```python
from build123d import *

# Parameters (mm, degrees)
SKETCH1_W           = 165
SKETCH1_H           = 107
BOSS_EXTRUDE1_DEPTH = 10
SKETCH2_W           = 9
SKETCH2_H           = 9
CUT_EXTRUDE1_DEPTH  = 5
SKETCH3_W           = 17.586391164
SKETCH3_H           = 24.095664715
CUT_EXTRUDE2_DEPTH  = 5
SKETCH6_W           = 10.5
SKETCH6_H           = 16
CUT_EXTRUDE3_DEPTH  = 130.934107916
SKETCH8_R           = 3.05
CUT_EXTRUDE4_DEPTH  = 130.934107916
SKETCH9_W           = 9
SKETCH9_H           = 9
CUT_EXTRUDE5_DEPTH  = 5


with BuildPart() as part:
    # Sketch1 → Boss-Extrude1 (new body)
    with BuildSketch(Plane.XY):
        with BuildLine():
            Line((-106.68, 73.5), (-31.75, 73.5))
            ThreePointArc((-31.75, 73.5), (0, 58.078932216), (31.75, 73.5))
            Line((31.75, 73.5), (106.68, 73.5))
            Line((106.68, 73.5), (97.79, -63.5))
            Line((97.79, -63.5), (-97.79, -63.5))
            Line((-97.79, -63.5), (-106.68, 73.5))
        make_face()
        Rectangle(SKETCH1_W, SKETCH1_H, mode=Mode.SUBTRACT)
    extrude(amount=BOSS_EXTRUDE1_DEPTH)

    # Sketch2 → Cut-Extrude1 (cut)
    with BuildSketch(Plane.XY.offset(10)):
        with Locations((78, 58)):
            Rectangle(SKETCH2_W, SKETCH2_H)
        with Locations((-78, 58)):
            Rectangle(SKETCH2_W, SKETCH2_H)
    extrude(amount=-CUT_EXTRUDE1_DEPTH, mode=Mode.SUBTRACT)

    # Sketch3 → Cut-Extrude2 (cut)
    with BuildSketch(Plane.XY.offset(10)):
        with Locations((-91.293195582, 41.716713566)):
            Rectangle(SKETCH3_W, SKETCH3_H)
    extrude(amount=-CUT_EXTRUDE2_DEPTH, mode=Mode.SUBTRACT)

    # Sketch6 → Cut-Extrude3 (cut, through all)
    with BuildSketch(Plane(origin=(0, 0, 0), x_dir=(-1, 0, 0), z_dir=(0, 0, -1))):
        with Locations((92.403067071, 12.157965544)):
            Rectangle(SKETCH6_W, SKETCH6_H)
    extrude(amount=-CUT_EXTRUDE3_DEPTH, mode=Mode.SUBTRACT)

    # Sketch8 → Cut-Extrude4 (cut, through all)
    with BuildSketch(Plane(origin=(0, 0, 0), x_dir=(-1, 0, 0), z_dir=(0, 0, -1))):
        with Locations((91.642033661, -12.875359706)):
            Circle(SKETCH8_R)
    extrude(amount=-CUT_EXTRUDE4_DEPTH, mode=Mode.SUBTRACT)

    # Sketch9 → Cut-Extrude5 (cut)
    with BuildSketch(Plane.XY.offset(10)):
        with Locations((78, -58)):
            Rectangle(SKETCH9_W, SKETCH9_H)
        with Locations((-78, -58)):
            Rectangle(SKETCH9_W, SKETCH9_H)
    extrude(amount=-CUT_EXTRUDE5_DEPTH, mode=Mode.SUBTRACT)


solid = part.part
```
Geometry: final body of the model. Coordinates: model frame, mm. A direction names the side the tool comes from. Round coordinates to 2 decimals unless told otherwise and drop trailing zeros. Write each loop counter-clockwise with the first axis right and the second up, starting at its lowest first coordinate (ties: lowest second). Pieces come first, ordered by that corner, then holes.
Item 1: Section query A-A (x = -77). Return loops of the section in (y, z), plus the area to 3 significant figures.
Item 2: Section query D-D (y = 43). Return loops of the section in (x, z), plus the area to 3 significant figures.
Item 3: Pin query (flat end, axial travel): P1, Ø1.5, axis at y = -58.5, z = 7, coming from the +X side; P2, Ø2.5, axis at y = -57.5, z = 7, coming from the -X side; P3, Ø4, axis at y = 3.5, z = 8, coming from the +X side. Return the tip coordinate at first contact, or that it passes through.
Item 4: Mould query, pull axis Y, two halves, no side actions, for faces 4 (the face through (-70, 73.5, 5)), 5 (the face through (1, -63.5, 5)), 6 (the face through (78, 58, 5)). Classes: +Y half, -Y half, draft (parallel to the pull), parting line (faces both ways), or undercut.
Item 5: Section query B-B (y = 17.5). Return loops of the section in (x, z), plus the area to 3 significant figures.
Item 6: Set-up query: faces 1 (the face through (-0.511, 58.082, 4.93)), 2 (the face through (-92, 20.158, 5)), 3 (the face through (-91, 53.765, 8)). Return all of +Z, -Z, +X, -X, +Y, -Y with unobstructed straight access to the full face (end or side cutting, diameter ignored); none if empty.
Item 7: Section query C-C (z = 2.5). Return loops of the section in (x, y), plus the area to 3 significant figures.
Item 8: Material intervals for L1, parallel to Y at x = 32.5, z = 5; L2, parallel to Y at x = -0.5, z = 7; L3, parallel to Y at x = -94, z = 6, sorted ascending.
Completed:
1. outline: (-63.5, 0) - (-53.5, 0) - (-53.5, 5) - (-62.5, 5) - (-62.5, 10) - (-63.5, 10) - close; (53.5, 0) - (73.5, 0) - (73.5, 10) - (62.5, 10) - (62.5, 5) - (53.5, 5) - close
1. area: 210 mm2
2. outline: (-104.7, 0) - (-82.5, 0) - (-82.5, 5) - (-100.09, 5) - (-100.09, 10) - (-104.7, 10) - close; (82.5, 0) - (104.7, 0) - (104.7, 10) - (82.5, 10) - close
2. area: 356 mm2
3. P1: stops at x = 98.16
3. P2: stops at x = -98.26
3. P3: stops at x = 102.27
4. face 4: +Y half
4. face 5: -Y half
4. face 6: undercut
5. outline: (-103.05, 0) - (-97.65, 0) - (-97.65, 10) - (-103.05, 10) - close; (-87.15, 0) - (-82.5, 0) - (-82.5, 10) - (-87.15, 10) - close; (82.5, 0) - (103.05, 0) - (103.05, 10) - (82.5, 10) - close
5. area: 306 mm2
6. face 1: +Z, -Z, +Y
6. face 2: +Z, -Z
6. face 3: +Z
7. outline: (-106.68, 73.5) - (-97.79, -63.5) - (97.79, -63.5) - (106.68, 73.5) - (31.75, 73.5) arc R40.4 cw to (-31.75, 73.5) - close; hole (-97.65, 4.16) - (-87.15, 4.16) - (-87.15, 20.16) - (-97.65, 20.16) - close; hole circle Ø6.1 at (-91.64, -12.88); hole (-82.5, -53.5) - (82.5, -53.5) - (82.5, 53.5) - (-82.5, 53.5) - close
7. area: 9,480 mm2
8. L1: y = -63.5 to -53.5, 53.5 to 73.5
8. L2: y = -63.5 to -53.5, 53.5 to 58.08
8. L3: y = -63.5 to -14.81, -10.94 to 4.16, 20.16 to 29.67, 53.76 to 73.5
